from build123d import *

# Parameters (mm, degrees)
F1_DEPTH = 12.7
F3_DEPTH = 31.75
F4_W     = 31.75
F4_H     = 14.224
F5_DEPTH = 31.75
F6_R     = 6.35
F7_DEPTH = 25.4


with BuildPart() as f1:
    # F0 (on Front) → F1 (new body)
    with BuildSketch(Plane.XZ):
        Polygon((-127, 0), (0, 0), (0, 22.098), (-47.498, 69.85), (-79.248, 69.85), (-127, 22.098), align=None)
    extrude(amount=F1_DEPTH)

    # F2 (on face) → F3 (join)
    with BuildSketch(Plane.XZ.offset(12.7)):
        Polygon((-31.5910821557, 0), (-31.5910821557, 12.7), (-50.6410821557, 31.75), (-76.0410821557, 31.75), (-95.0910821557, 12.7), (-95.0910821557, 0), align=None)
    extrude(amount=F3_DEPTH)

    # F4 (on face) → F5 (join)
    with BuildSketch(Plane.XZ.offset(12.7)):
        with Locations((-63.373, 62.738)):
            Rectangle(F4_W, F4_H)
    extrude(amount=F5_DEPTH)

    # F6 (on face) → F7 (cut)
    with BuildSketch(Plane.XY.offset(69.85)):
        with Locations((-64.1456767917, -28.702)):
            Circle(F6_R)
    extrude(amount=-F7_DEPTH, mode=Mode.SUBTRACT)


solid = f1.part
The listing builds one solid part. Answer for the finished solid, in the listing's coordinates (mm). A direction names the side the tool comes from. Coordinates: 2 decimals unless noted, no trailing zeros. Write each loop counter-clockwise with the first axis right and the second up, starting at its lowest first coordinate (ties: lowest second). Pieces come first, ordered by that corner, then holes. Notation, with made-up numbers: (-34.5, -22) -> (-2.5, -22) arc R26 cw to (-2.5, -3) -> close; hole circle Ø11 at (85.25, 29). An arc over 180 degrees is marked (long way). One line per question, with ' | ' between items.
1. Which of the six approach directions +Z, -Z, +X, -X, +Y, -Y give full straight-line access (tool end or side, diameter ignored) to faces 5 (the flat face through (-79.248, -28, 63)), 6 (the flat face through (-95.091, -28, 6)), 7 (the flat face through (-63, -28, 31.75)), 8 (the flat face through (-31.591, -28, 6))?
Verdict:
face 5: +Z, -X, -Y | face 6: +Z, -Z, -X, -Y | face 7: +X, -X, -Y | face 8: +Z, -Z, +X, -Y
2. Straight lines are drawn through the part: line 1 (Z direction, x = -51, y = -15); line 2 (Y direction, x = -69, z = 32); line 3 (Z direction, x = -66, y = -34). For each, find the intervals that lie inside material, in ascending order.
Verdict:
line 1: z = 0 to 31.75, 55.63 to 69.85 | line 2: y = -12.7 to 0 | line 3: z = 0 to 31.75
3. Given pin 1 Ø7 at (y, z) = (-21.5, 62.5) entering from +X; pin 2 Ø12 at (x, y) = (-47.5, -33) entering from -Z; pin 3 Ø1.5 at (x, z) = (-19.5, 22.5) entering from -Y; pin 4 Ø6.5 at (y, z) = (-33, 8.5) entering from +X, each flat-ended and moving along its own axis, determine where each tip first touches the part or whether it passes through.
Verdict:
pin 1: stops at x = -47.5 | pin 2: stops at z = 0 | pin 3: stops at y = -12.7 | pin 4: stops at x = -31.59
4. Section B-B (z = 5) is taken. Determine the outline of the cut face in (x, y), and give its area (3 significant figures).
Verdict:
outline: (-127, -12.7) -> (-95.09, -12.7) -> (-95.09, -44.45) -> (-31.59, -44.45) -> (-31.59, -12.7) -> (0, -12.7) -> (0, 0) -> (-127, 0) -> close | area: 3,630 mm^2
5. Section D-D (x = -69) is taken. Determine the outline of the cut face in (y, z).
Verdict:
outline: (-44.45, 0) -> (0, 0) -> (0, 69.85) -> (-24.61, 69.85) -> (-24.61, 55.63) -> (-12.7, 55.63) -> (-12.7, 31.75) -> (-44.45, 31.75) -> close; (-44.45, 55.63) -> (-32.8, 55.63) -> (-32.8, 69.85) -> (-44.45, 69.85) -> close
6. For a pull along Y with two mould halves and no side action, classify faces 1 (the flat face through (-64, 0, 28)), 2 (the flat face through (-85.43, -28.35, 22.36)), 3 (the flat face through (-64, -44.45, 63)), 4 (the cylindrical face through (-58.09, -26.79, 62.84)) as released by +Y, released by -Y, zero draft, split by the parting line, or undercut.
Verdict:
face 1: released by +Y | face 2: zero draft | face 3: released by -Y | face 4: undercut
7. Section C-C (y = -25) is taken. Determine the outline of the cut face in (x, z), and give its area (3 significant figures).
Verdict:
outline: (-95.09, 0) -> (-31.59, 0) -> (-31.59, 12.7) -> (-50.64, 31.75) -> (-76.04, 31.75) -> (-95.09, 12.7) -> close; (-79.25, 55.63) -> (-69.3, 55.63) -> (-69.3, 69.85) -> (-79.25, 69.85) -> close; (-58.99, 55.63) -> (-47.5, 55.63) -> (-47.5, 69.85) -> (-58.99, 69.85) -> close | area: 1,960 mm^2
8. Section A-A (y = -15.5) is taken. Determine the outline of the cut face in (x, z).
Verdict:
outline: (-95.09, 0) -> (-31.59, 0) -> (-31.59, 12.7) -> (-50.64, 31.75) -> (-76.04, 31.75) -> (-95.09, 12.7) -> close; (-79.25, 55.63) -> (-47.5, 55.63) -> (-47.5, 69.85) -> (-79.25, 69.85) -> close
